Work out the finished part from the listing and answer in its coordinate system (mm). Face numbers are marked on the shaded views. A direction names the side the tool comes from. Give positions to 0.01 mm unless a question says otherwise; leave off trailing zeros. Loops run counter-clockwise (first coordinate to the right, second up) from the corner with the lowest first, then second, coordinate; pieces in that order, holes last. Notation, with made-up numbers: (45.5, 3.5) -> (100.5, 3.5) arc R32 cw to (100.5, 40.5) -> close; hole circle Ø10 at (43, -25). An arc over 180 degrees is marked (long way). Answer as CSV lines item,"result". Start each with the question number.
1. Find section B-B, the plane x = 16.5. Give the vertices of the cut face in (y, z), and give its area (3 significant figures).
2. Find section D-D, the plane y = -270. Give the vertices of the cut face in (x, z), and give its area (3 significant figures).
3. Determine the mould class of the marked faces 3, 4 and 5 for opening direction Z: +Z half, -Z half, draft (parallel to the pull), parting line (faces both ways), or undercut.
4. Find section C-C, the plane y = -329.5. Give the vertices of the cut face in (x, z), and give its area (3 significant figures).
5. Find section A-A, the plane z = 0. Give the vertices of the cut face in (x, y).
6. A tool of negligible diameter and unlimited length cuts with its end or side. For the marked faces 1 and 2, from which of +Z, -Z, +X, -X, +Y, -Y can it reach the whole face along a straight path? Write none if from no direction.
7. Find the intervals of material crossed by line 1 along Y through (x, z) = (24, 0); line 2 along Z through (x, y) = (-15, -178); line 3 along Z through (x, y) = (23.8, -155), in increasing order.
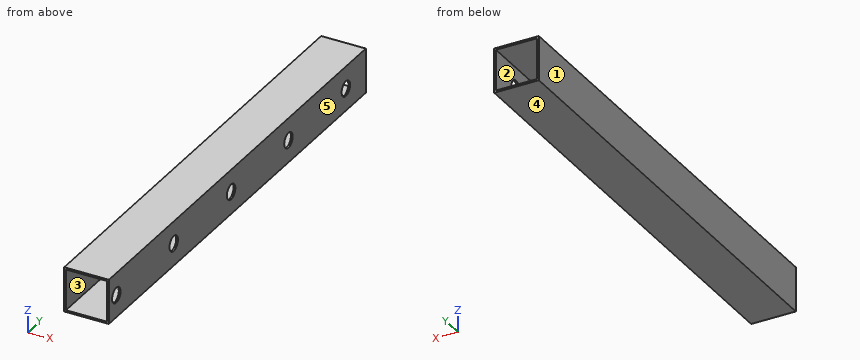
Autodesk Inventor part; units mm, degrees
ref_plane "YZ Plane" through (0, 0, 0) normal (1, 0, 0) x (0, 1, 0)
ref_plane "XZ Plane" through (0, 0, 0) normal (0, 1, 0) x (-1, 0, 0)
ref_plane "XY Plane" through (0, 0, 0) normal (0, 0, 1) x (1, 0, 0)
sketch "Sketch9" plane through (0, 0, 0) normal (0, 1, 0) x (-1, 0, 0)
  line L0 (25, 25) -> (-25, 25)
  line L1 (-25, 25) -> (-25, -25)
  line L2 (-25, -25) -> (25, -25)
  line L3 (25, -25) -> (25, 25)
  line L4 (25, 25) -> (-25, -25) construction
  line L5 (-25, 25) -> (25, -25) construction
  line L6 (-23, 23) -> (23, 23)
  line L7 (23, 23) -> (23, -23)
  line L8 (23, -23) -> (-23, -23)
  line L9 (-23, -23) -> (-23, 23)
  point P0 (0, 0)
  dimension "d172" = 50
  dimension "d173" = 50
  dimension "d174" = 2
extrude "Extrusion3" add sketch "Sketch9" against normal blind 515
sketch "Sketch10" plane through (0, 0, 0) normal (1, 0, 0) x (0, 1, 0)
  line L0 (0, 25) -> (0, -25) construction
  line L1 (0, 25) -> (-515, 25) construction
  line L2 (-515, -25) -> (-515, 25) construction
  line L3 (0, -25) -> (-515, -25) construction
  line L4 (-48.5, 8.5) -> (-31.5, 8.5)
  line L5 (-31.5, 8.5) -> (-31.5, -8.5)
  line L6 (-31.5, -8.5) -> (-48.5, -8.5)
  line L7 (-48.5, -8.5) -> (-48.5, 8.5)
  line L8 (-48.5, 8.5) -> (-31.5, -8.5) construction
  line L9 (-31.5, 8.5) -> (-48.5, -8.5) construction
  line L10 (-163.5, 8.5) -> (-146.5, 8.5)
  line L11 (-146.5, 8.5) -> (-146.5, -8.5)
  line L12 (-146.5, -8.5) -> (-163.5, -8.5)
  line L13 (-163.5, -8.5) -> (-163.5, 8.5)
  line L14 (-163.5, 8.5) -> (-146.5, -8.5) construction
  line L15 (-146.5, 8.5) -> (-163.5, -8.5) construction
  line L16 (-278.5, 8.5) -> (-261.5, 8.5)
  line L17 (-261.5, 8.5) -> (-261.5, -8.5)
  line L18 (-261.5, -8.5) -> (-278.5, -8.5)
  line L19 (-278.5, -8.5) -> (-278.5, 8.5)
  line L20 (-278.5, 8.5) -> (-261.5, -8.5) construction
  line L21 (-261.5, 8.5) -> (-278.5, -8.5) construction
  circle A0 centre (-500, 0) radius 8.5
  line L22 (0, 0) -> (40, 0)
  circle A1 centre (-40, 0) radius 8.5
  circle A2 centre (-155, 0) radius 8.5
  circle A3 centre (-270, 0) radius 8.5
  line L23 (-376.5, -8.5) -> (-393.5, -8.5)
  line L24 (-393.5, -8.5) -> (-393.5, 8.5)
  line L25 (-393.5, 8.5) -> (-376.5, 8.5)
  line L26 (-376.5, 8.5) -> (-376.5, -8.5)
  line L27 (-376.5, -8.5) -> (-393.5, 8.5) construction
  line L28 (-393.5, -8.5) -> (-376.5, 8.5) construction
  circle A4 centre (-385, 0) radius 8.5
  dimension "d177" = 17
  dimension "d178" = 17
  dimension "d181" = 40
  dimension "d182" = 80
  dimension "d185" = 540
  dimension "d186" = 17
  dimension "d188" = 460
  dimension "d189" = 115
  dimension "d190" = 115
  dimension "d191" = 115
extrude "Extrusion4" cut sketch "Sketch10" along normal through all contours A1 | A2 | A3 | A0 | A4
properties part number "TKS 3511 FDS way tube 7" material "Stainless Steel"
Resolved:
1,outline,"(-515, -25) -> (0, -25) -> (0, -23) -> (-515, -23) -> close; (-515, 23) -> (0, 23) -> (0, 25) -> (-515, 25) -> close"
1,area,"2,060 mm^2"
2,outline,"(-25, -25) -> (25, -25) -> (25, -8.5) -> (23, -8.5) -> (23, -23) -> (-23, -23) -> (-23, 23) -> (23, 23) -> (23, 8.5) -> (25, 8.5) -> (25, 25) -> (-25, 25) -> close"
2,area,"350 mm^2"
3,face 3,"undercut"
3,face 4,"-Z half"
3,face 5,"draft"
4,outline,"(-25, -25) -> (25, -25) -> (25, 25) -> (-25, 25) -> close; hole (-23, -23) -> (23, -23) -> (23, 23) -> (-23, 23) -> close"
4,area,"384 mm^2"
5,outline,"(-25, -515) -> (-23, -515) -> (-23, 0) -> (-25, 0) -> close; (23, -515) -> (25, -515) -> (25, -508.5) -> (23, -508.5) -> close; (23, -491.5) -> (25, -491.5) -> (25, -393.5) -> (23, -393.5) -> close; (23, -376.5) -> (25, -376.5) -> (25, -278.5) -> (23, -278.5) -> close; (23, -261.5) -> (25, -261.5) -> (25, -163.5) -> (23, -163.5) -> close; (23, -146.5) -> (25, -146.5) -> (25, -48.5) -> (23, -48.5) -> close; (23, -31.5) -> (25, -31.5) -> (25, 0) -> (23, 0) -> close"
6,face 1,"+Z, -Z, -X, +Y, -Y"
6,face 2,"+Y, -Y"
7,line 1,"y = -515 to -508.5, -491.5 to -393.5, -376.5 to -278.5, -261.5 to -163.5, -146.5 to -48.5, -31.5 to 0"
7,line 2,"z = -25 to -23, 23 to 25"
7,line 3,"z = -25 to -8.5, 8.5 to 25"
